Input: part model. Units: mm. Frame: model coordinates. A direction names the side the tool comes from. Give positions to 0.01 mm unless a question says otherwise; leave off trailing zeros. Order: outer loops, then holes, each group sorted by start corner. A loop starts at its lowest first (then second) coordinate and runs counter-clockwise, first axis right, second up. Notation, with made-up numbers: (-20, -0.5) - (7, -0.5) arc R24 cw to (7, 20.5) - close; hole circle Ø3 at (6, 13.25). An arc over 180 degrees is marked (long way). Answer in a Markdown table with one row per item. Add a question column.
1. Mould query, pull axis Y, two halves, no side actions, for faces 1 (the face through (-20.81, -17.11, 2.36)), 2 (the face through (-18.84, -27.02, 1.36)), 3 (the face through (-18.835, 4.376, 16.742)). Classes: released by +Y, released by -Y, zero draft, split by the parting line, or undercut.
2. Section query C-C on z = -1. Return loops of the section in (x, y).
3. Section query A-A on y = 0. Return loops of the section in (x, z), and give its area (3 significant figures).
4. Section query B-B on z = -6.5. Return loops of the section in (x, y), and give its area (3 significant figures).
5. Ray query, line 1 (Y direction, x = -18.15, z = 20); line 2 (Y direction, x = -19.65, z = 25.5); line 3 (Z direction, x = -18.75, y = -46.5). Return the intervals inside material, ascending. Write a range as [from, to].
6. Section query D-D on x = -19.5. Return loops of the section in (y, z).
7. Access query for faces 4 (the face through (-20.3, -14.4, 0.3)), 5 (the face through (-18.84, -56.22, 23)). Directions: +Z, -Z, +X, -X, +Y, -Y. A direction counts if a zero-diameter tool reaches every point of the face in a straight line with its end or side. Return the directions, or none.
8. Contact query for flat-ended pins moving along their axis: pin 1 (1.5 mm diameter, centred on x = -19.5, y = -40.5, fed in from -Z); pin 2 (13 mm diameter, centred on y = 0, z = 0, fed in from -X); pin 3 (4 mm diameter, centred on y = -14.55, z = -1.59, fed in from -X); pin 4 (2 mm diameter, centred on x = -19, y = -36, fed in from +Z). Output: stop coordinate, or through.
```python
from build123d import *

# Parameters (mm, degrees)
BOSS_EXTRUDE1_START  = -11.3
SKETCH2_R            = 8
BOSS_EXTRUDE1_DEPTH  = 5
BOSS_EXTRUDE2_START  = -11.3
BOSS_EXTRUDE2_DEPTH  = 5
CUT_EXTRUDE2_START   = -11.3
CUT_EXTRUDE2_DEPTH   = 1
M3_CLEARANCE_HOLE1_D = 3.2
M3_CLEARANCE_HOLE2_D = 3.2


# Read off the part's stored shape, not the designer's step: Intersect1
with BuildPart() as part:
    # Sketch2 → Boss-Extrude1 (new body)
    with BuildSketch(Plane(origin=(0, 0, 0), x_dir=(0, 0, -1), z_dir=(1, 0, 0)).offset(BOSS_EXTRUDE1_START)):
        with BuildLine():
            Line((9.0940801, -4.15905123), (-12.117081171, -50.538859741))
            ThreePointArc((-12.117081171, -50.538859741), (-25.370212501, -55.473888611), (-30.305241372, -42.220757281))
            Line((-30.305241372, -42.220757281), (-9.0940801, 4.15905123))
            ThreePointArc((-9.0940801, 4.15905123), (4.15905123, 9.0940801), (9.0940801, -4.15905123))
        make_face()
        with Locations((-21.211161271, -46.379808511)):
            Circle(SKETCH2_R, mode=Mode.SUBTRACT)
        Circle(SKETCH2_R, mode=Mode.SUBTRACT)
    boss_extrude1 = extrude(amount=-BOSS_EXTRUDE1_DEPTH)

    # Sketch2<3> → Boss-Extrude2 (add)
    with BuildSketch(Plane(origin=(0, 0, 0), x_dir=(0, 0, -1), z_dir=(1, 0, 0)).offset(BOSS_EXTRUDE2_START)):
        with BuildLine():
            ThreePointArc((-9.0940801, 4.15905123), (-6.824825213, 7.309019141), (-3.526945256, 9.357385167))
            Line((-3.526945256, 9.357385167), (-30.332118628, -0.745905163))
            ThreePointArc((-30.332118628, -0.745905163), (-32.00821012, -2.077061023), (-32.595823612, -4.135208005))
            Line((-32.595823612, -4.135208005), (-31.205835053, -46.706145748))
            ThreePointArc((-31.205835053, -46.706145748), (-31.015487287, -44.411257932), (-30.305241372, -42.220757281))
            Line((-30.305241372, -42.220757281), (-9.0940801, 4.15905123))
        make_face()
    boss_extrude2 = extrude(amount=-BOSS_EXTRUDE2_DEPTH)

    # Sketch2<6> → Cut-Extrude2 (cut)
    with BuildSketch(Plane(origin=(0, 0, 0), x_dir=(0, 0, -1), z_dir=(1, 0, 0)).offset(CUT_EXTRUDE2_START)):
        with BuildLine():
            Line((2.200817213, -19.231691933), (5.528058196, -11.956427853))
            Line((5.528058196, -11.956427853), (3.553212429, -11.053259569))
            ThreePointArc((3.553212429, -11.053259569), (0.981018146, -9.876902238), (-0.195339185, -12.449096521))
            Line((-0.195339185, -12.449096521), (-1.169865506, -14.579972035))
            ThreePointArc((-1.169865506, -14.579972035), (-2.346222837, -17.152166318), (0.225971446, -18.328523649))
            Line((0.225971446, -18.328523649), (2.200817213, -19.231691933))
        make_face()
    cut_extrude2 = extrude(amount=-CUT_EXTRUDE2_DEPTH, mode=Mode.SUBTRACT)

    # M3 Clearance Hole1 (through all)
    with Locations(Plane(origin=(-11.3, 0, 0), x_dir=(0, 0, 1), z_dir=(1, 0, 0))):
        with Locations((29.097687789, 4.020989972)):
            m3_clearance_hole1 = Hole(M3_CLEARANCE_HOLE1_D / 2)

    # M3 Clearance Hole2 (through all)
    with Locations(Plane.ZY.offset(16.3)):
        with Locations((-1.590917679, -14.554297085)):
            m3_clearance_hole2 = Hole(M3_CLEARANCE_HOLE2_D / 2)

    # Mirror2: Boss-Extrude1, Boss-Extrude2, Cut-Extrude2, M3 Clearance Hole1, M3 Clearance Hole2 across plane
    add(boss_extrude1.mirror(Plane.ZY.offset(16.3)))
    add(boss_extrude2.mirror(Plane.ZY.offset(16.3)))
    add(cut_extrude2.mirror(Plane.ZY.offset(16.3)), mode=Mode.SUBTRACT)
    add(m3_clearance_hole1.mirror(Plane.ZY.offset(16.3)), mode=Mode.SUBTRACT)
    add(m3_clearance_hole2.mirror(Plane.ZY.offset(16.3)), mode=Mode.SUBTRACT)


with BuildPart() as body_2:
    # Intersect1: the piece on the far side of the plane
    add(part.part)
    split(bisect_by=Plane.YZ.offset(-16.3), keep=Keep.BOTTOM)


with BuildPart() as part_1:
    add(part.part)

    # Intersect1
    split(bisect_by=Plane.YZ.offset(-16.3), keep=Keep.TOP)


solid = body_2.part
```
Answer:
| question | item | result |
|---|---|---|
| 1 | face 1 | undercut |
| 1 | face 2 | released by -Y |
| 1 | face 3 | released by +Y |
| 2 | outline | (-21.3, -21.86) - (-16.3, -21.86) - (-16.3, -16.04) - (-20.3, -16.04) - (-20.3, -18.68) - (-21.3, -18.68) - close; (-21.3, -9.87) - (-20.3, -9.87) - (-20.3, -13.07) - (-16.3, -13.07) - (-16.3, -7.94) - (-21.3, -7.94) - close; (-21.3, 7.94) - (-16.3, 7.94) - (-16.3, 9.95) - (-21.3, 9.95) - close |
| 3 | outline | (-21.3, -10) - (-16.3, -10) - (-16.3, -8) - (-21.3, -8) - close; (-21.3, 8) - (-16.3, 8) - (-16.3, 28.35) - (-21.3, 28.35) - close |
| 3 | area | 112 mm² |
| 4 | outline | (-21.3, -9.83) - (-16.3, -9.83) - (-16.3, -4.66) - (-21.3, -4.66) - close; (-21.3, 4.66) - (-16.3, 4.66) - (-16.3, 7.6) - (-21.3, 7.6) - close |
| 4 | area | 40.5 mm² |
| 5 | line 1 | y = [-56.31, -54.29], [-38.47, 3.15] |
| 5 | line 2 | y = [-55.41, -53.13], [-39.63, 1.08] |
| 5 | line 3 | z = [10.27, 13.21], [29.21, 31.21] |
| 6 | outline | (-50.54, 12.12) - (-4.16, -9.09) arc R10 ccw to (9.36, 3.53) - (-0.75, 30.33) arc R3.5 ccw to (-4.14, 32.6) - (-46.71, 31.21) arc R10 ccw to start; hole circle Ø16 at (-46.38, 21.21); hole circle Ø3.2 at (-14.55, -1.59); hole circle Ø16 at (0, 0); hole circle Ø3.2 at (-4.02, 29.1) |
| 7 | face 4 | -X |
| 7 | face 5 | +X, -X, -Y |
| 8 | pin 1 | stops at z = 7.18 |
| 8 | pin 2 | passes through |
| 8 | pin 3 | stops at x = -20.3 |
| 8 | pin 4 | stops at z = 31.59 |
